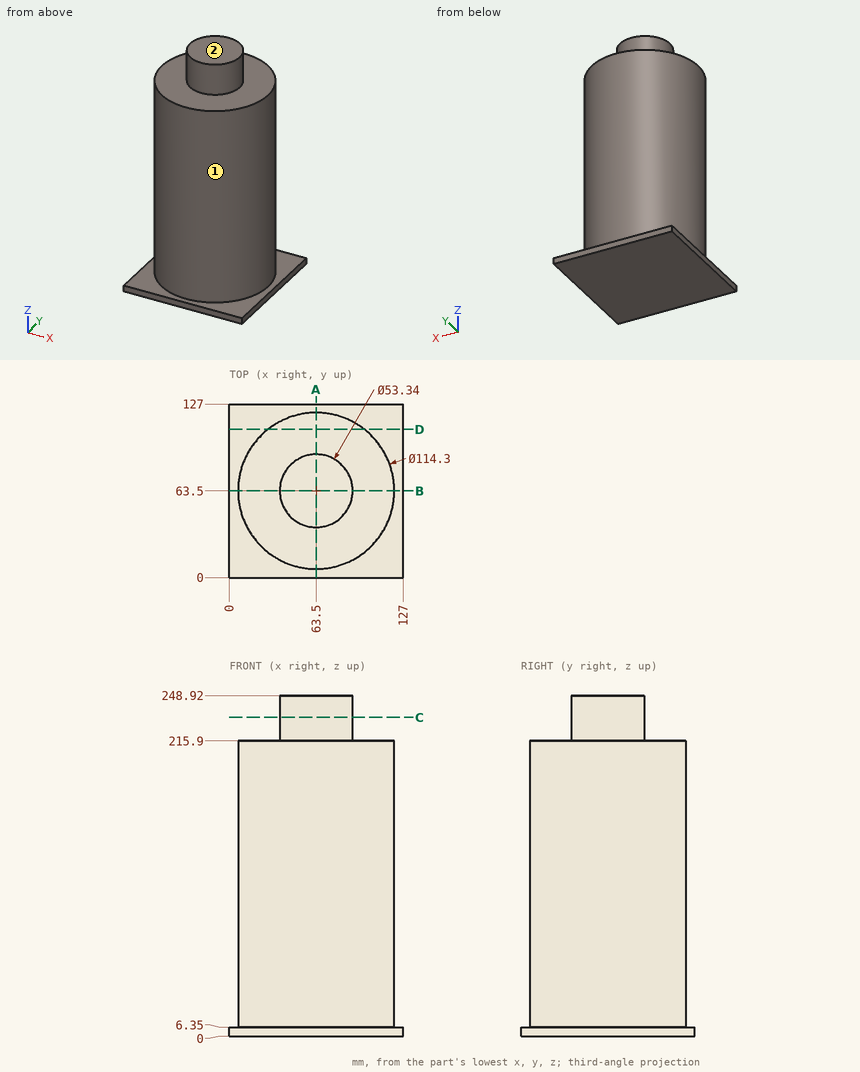
For this review, use the dimensioned drawing (mm, ordinates from the lowest corner) and the shaded views. A direction names the side the tool comes from. Coordinates: 2 decimals unless noted, no trailing zeros. Loops run counter-clockwise (first coordinate to the right, second up) from the corner with the lowest first, then second, coordinate; pieces in that order, holes last. Notation, with made-up numbers: (-15, 34) -> (9, 34) arc R27 ccw to (9, 54) -> close; hole circle Ø2 at (20.25, 80). An arc over 180 degrees is marked (long way). Use a Markdown table: item, result. Add a question column.
Item 1: We need section A-A, the plane x = 63.5. Write out the cut boundary in (y, z), and give its area (3 significant figures).
Item 2: Wall thickness on L1, parallel to Z at x = 36, y = 74.5; L2, parallel to Z at x = 41, y = 122.5; L3, parallel to X at y = 61, z = 153: over which ranges is each line inside the solid? List them lowest first. Write a range as from..to.
Item 3: We need section C-C, the plane z = 233. Write out the cut boundary in (x, y), and give its area (3 significant figures).
Item 4: We need section D-D, the plane y = 108.5. Write out the cut boundary in (x, z).
Item 5: Clearance check with flat-ended pins moving along their axes: P1, Ø2, axis at x = 54, z = 77, coming from the +Y side; P2, Ø6, axis at x = 99, y = 114, coming from the -Z side; P3, Ø1, axis at x = 95.5, z = 197, coming from the +Y side; P4, Ø6, axis at x = 68, z = 114.5, coming from the -Y side. State where each tip first meets the part, or that it passes through.
Item 6: Machinability: for the marked faces 1 and 2, which of the approach directions +Z, -Z, +X, -X, +Y, -Y give a long, thin tool a straight path to every point of the face, cutting with its end or side? Answer none if there is none.
Numbers:
| question | item | result |
|---|---|---|
| 1 | outline | (0, 0) -> (127, 0) -> (127, 6.35) -> (120.65, 6.35) -> (120.65, 215.9) -> (90.17, 215.9) -> (90.17, 248.92) -> (36.83, 248.92) -> (36.83, 215.9) -> (6.35, 215.9) -> (6.35, 6.35) -> (0, 6.35) -> close |
| 1 | area | 26,500 mm^2 |
| 2 | L1 | z = 0..215.9 |
| 2 | L2 | z = 0..6.35 |
| 2 | L3 | x = 6.4..120.6 |
| 3 | outline | circle Ø53.34 at (63.5, 63.5) |
| 3 | area | 2,230 mm^2 |
| 4 | outline | (0, 0) -> (127, 0) -> (127, 6.35) -> (98.73, 6.35) -> (98.73, 215.9) -> (28.27, 215.9) -> (28.27, 6.35) -> (0, 6.35) -> close |
| 5 | P1 | stops at y = 120.01 |
| 5 | P2 | stops at z = 0 |
| 5 | P3 | stops at y = 111.19 |
| 5 | P4 | stops at y = 6.37 |
| 6 | face 1 | +Z |
| 6 | face 2 | +Z, +X, -X, +Y, -Y |
